Verification items for this drawing (mm, ordinates from the low corner). Round coordinates to 2 decimals unless told otherwise and drop trailing zeros. Answer in a Markdown table with one row per item. Add a question column.
1. Draft check along Z on the marked faces 1, 2 and 3. Enter one of: +Z half, -Z half, draft (parallel to the pull), parting line (faces both ways), or undercut.
2. Depth check by flat-ended pin: P1, Ø3, axis at x = 20.64, z = 4.76, coming from the +Y side; P2, Ø1.5, axis at x = 14, y = 3.5, coming from the -Z side (1 decimal); P3, Ø2, axis at y = 4, z = 45, coming from the +X side (1 decimal); P4, Ø1, axis at x = 37, y = 2, coming from the +Z side. Enter the tip coordinate at first touch or a pass-through.
3. Sectioned sample at C-C, the plane x = 19.5. Count the separate pieces of the cut face and the enclosed holes in it, then the cut area to 3 significant figures.
4. Material ranges on L1, parallel to Z at x = 20, y = 3.25 (1 decimal); L2, parallel to Z at x = 19.5, y = 0.5 (1 decimal); L3, parallel to X at y = 5.75, z = 30.5, recorded low to high. Write a range as from..to.
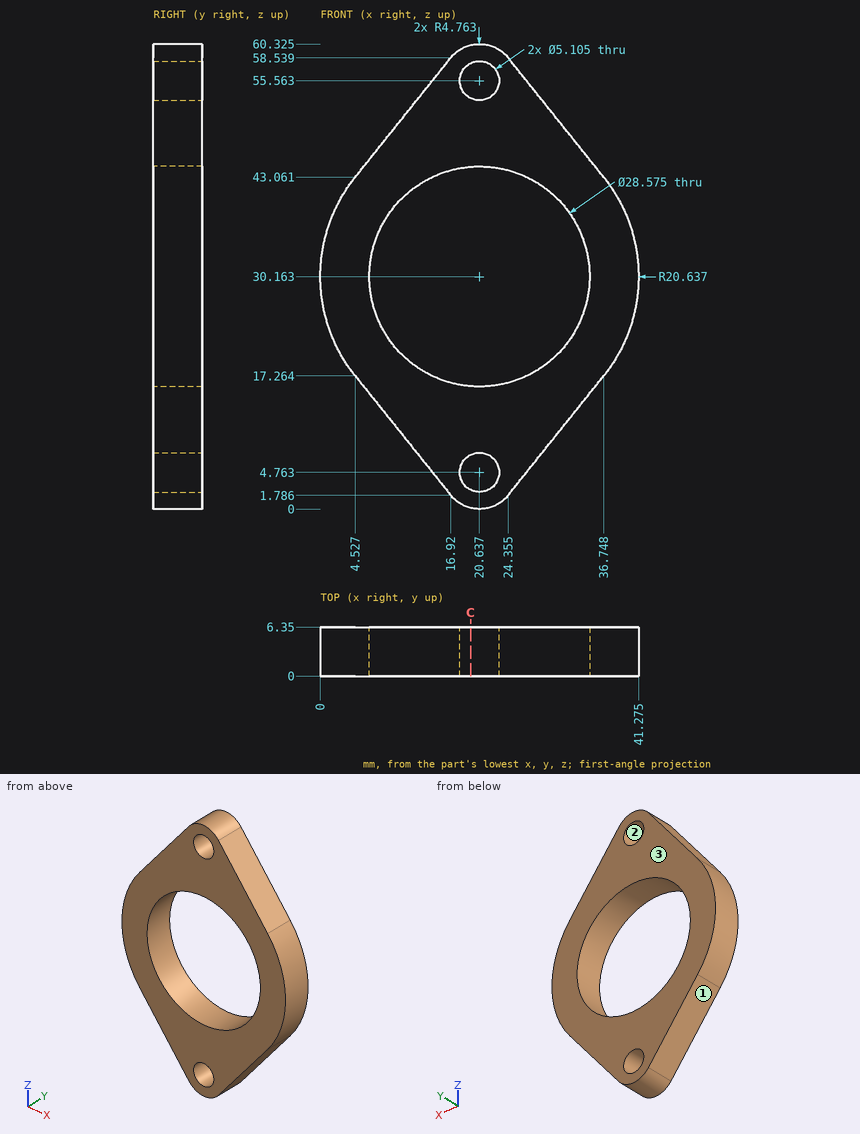
Answer key:
| question | item | result |
|---|---|---|
| 1 | face 1 | -Z half |
| 1 | face 2 | undercut |
| 1 | face 3 | draft |
| 2 | P1 | passes through |
| 2 | P2 | stops at z = 4.5 |
| 2 | P3 | stops at x = 36 |
| 2 | P4 | stops at z = 43.37 |
| 3 | separate pieces | 4 |
| 3 | enclosed holes | 0 |
| 3 | area | 142 mm² |
| 4 | L1 | z = 0..2.3, 7.2..15.9, 44.4..53.1, 58..60.3 |
| 4 | L2 | z = 0.1..2.5, 7..15.9, 44.4..53.3, 57.8..60.2 |
| 4 | L3 | x = 0..6.35, 34.92..41.27 |
